Source: CAD feature listing. Evaluate the final solid. Frame: model axes, mm. A direction names the side the tool comes from. Round coordinates to 2 decimals unless told otherwise and drop trailing zeros. Order: outer loops, then holes, each group sorted by start corner. A loop starts at its lowest first (then second) coordinate and runs counter-clockwise, first axis right, second up. Notation, with made-up numbers: (59.5, 66) - (78.5, 66) arc R15 cw to (78.5, 84) - close; hole circle Ø11 at (50, 31.25). An arc over 180 degrees is marked (long way). Put each result on its own line as item: value. Start each with the question number.
1) Mould query, pull axis X, two halves, no side actions, for faces 3 (the face through (9.53, -148.7, -0.14)), 4 (the face through (13, -301.625, 0)), 5 (the face through (-0.69, -148.7, 15.8)). Classes: +X half, -X half, draft (parallel to the pull), parting line (faces both ways), or undercut.
2) Section C-C on y = -32.5. Output: boundary loops of the cut face in (x, z) (3 decimals).
3) Section A-A on x = 0. Output: boundary loops of the cut face in (y, z) (3 decimals), then the cut area to 3 significant figures.
4) Contact query for flat-ended pins moving along their axis: P1, Ø8, axis at y = -207, z = 9, coming from the +X side (3 decimals); P2, Ø12, axis at x = 8.5, y = -114.5, coming from the +Z side; P3, Ø11.5, axis at x = 1, z = 5, coming from the -Y side (3 decimals); P4, Ø5, axis at x = -14, y = -95.5, coming from the -Z side (3 decimals). Output: stop coordinate, or through.
5) Line query: probe 1 along Z at (x, y) = (-6, 2); probe 2 along Z at (x, y) = (0, 1) (3 decimals); probe 3 along X at (y, z) = (-237, -13). Output: solid intervals per line, ascending. Write a range as [from, to].
6) Section B-B on x = -12.7. Output: boundary loops of the cut face in (y, z) (3 decimals).
7) Access query for faces 1 (the face through (-9.67, -148.7, -0.95)), 2 (the face through (0, -301.625, 13)). Directions: +Z, -Z, +X, -X, +Y, -Y. A direction counts if a zero-diameter tool reaches every point of the face in a straight line with its end or side. Return the directions, or none.
Autodesk Inventor part; units mm, degrees
ref_plane "YZ Plane" through (0, 0, 0) normal (1, 0, 0) x (0, 1, 0)
ref_plane "XZ Plane" through (0, 0, 0) normal (0, 1, 0) x (-1, 0, 0)
ref_plane "XY Plane" through (0, 0, 0) normal (0, 0, 1) x (1, 0, 0)
sketch "Sketch1" plane through (0, 0, 0) normal (0, 1, 0) x (-1, 0, 0)
  line L0 (19.05, 19.05) -> (-19.05, 19.05)
  line L1 (-19.05, 19.05) -> (-19.05, -19.05)
  line L2 (-19.05, -19.05) -> (19.05, -19.05)
  line L3 (19.05, -19.05) -> (19.05, 19.05)
  point P0 (0, 0)
  dimension "d0" = 38.1
  dimension "d1" = 38.1
  dimension "d77" = 19.05
  dimension "d78" = 19.05
extrude "Extrusion1" add sketch "Sketch1" along normal blind 3.175
hole "Hole5" at (-6.35, 3.175, -7.1374) direction (0, -1, 0) diameter 2.54 depth 3.175
hole "Hole6" at (6.35, 3.175, 7.1437) direction (0, -1, 0) diameter 2.54 depth 3.175
sketch "Sketch2" plane through (0, 3.175, 0) normal (0, 1, 0) x (1, 0, 0)
  circle A0 centre (0, 0) radius 3.175
  dimension "d58" = 6.35
extrude "Extrusion2" cut sketch "Sketch2" against normal blind 304.8
sketch "Sketch7" plane through (0, 3.175, 0) normal (0, 1, 0) x (1, 0, 0)
  circle A0 centre (0, 0) radius 19.05
  circle A1 centre (0, 12.7) radius 3.175
  circle A2 centre (0, 0) radius 12.7
  circle A3 centre (0, 0) radius 3.175
  circle A4 centre (-12.7, 0) radius 3.175
  circle A5 centre (0, -12.7) radius 3.175
  circle A6 centre (12.7, 0) radius 3.175
  dimension "d71" = 38.1
  dimension "d72" = 6.35
  dimension "d73" = 25.4
  dimension "d74" = 12.7
  dimension "d75" = 6.35
  dimension "d76" = 360
extrude "Extrusion7" add sketch "Sketch7" against normal blind 304.8 contours A1 A2 | A2 A1 | A4 A2 | A2 A4 | A6 A2 | A2 A6 | A5 A2 | A2 A5
properties part number "Shield_1"
Answer sheet:
1. face 3: undercut
1. face 4: draft
1. face 5: parting line
2. outline: circle Ø6.35 at (-12.7, 0); circle Ø6.35 at (0, -12.7); circle Ø6.35 at (0, 12.7); circle Ø6.35 at (12.7, 0)
3. outline: (-301.625, -15.875) - (0, -15.875) - (0, -19.05) - (3.175, -19.05) - (3.175, -3.175) - (0, -3.175) - (0, -9.525) - (-301.625, -9.525) - close; (-301.625, 9.525) - (0, 9.525) - (0, 3.175) - (3.175, 3.175) - (3.175, 19.05) - (0, 19.05) - (0, 15.875) - (-301.625, 15.875) - close
3. area: 3,930 mm^2
4. P1: x = 3.175
4. P2: z = 14.66
4. P3: y = -301.625
4. P4: z = -3.175
5. probe 1: [-19.05, -8.36], [-5.92, 19.05]
5. probe 2: [-19.05, -3.175], [3.175, 19.05]
5. probe 3: [-3.16, 3.16]
6. outline: (-301.625, -3.175) - (0, -3.175) - (0, -19.05) - (3.175, -19.05) - (3.175, 19.05) - (0, 19.05) - (0, 3.175) - (-301.625, 3.175) - close
7. face 1: -Y
7. face 2: +Z, -Z, +X, -X, -Y
